```python
from build123d import *

# Parameters (mm, degrees)
PAD_DEPTH    = 20
SKETCH001_R  = 1.8
POCKET_DEPTH = 29.501


with BuildPart() as part:
    # Sketch → Pad (new body)
    with BuildSketch(Plane.XY):
        with BuildLine():
            ThreePointArc((-2.5, 17.825543), (0, -18), (2.5, 17.825543))
            Line((2.5, 32.062411), (2.5, 17.825543))
            Line((6.5, 32.062411), (2.5, 32.062411))
            Line((6.5, 22.062411), (6.5, 32.062411))
            ThreePointArc((-6.5, 22.062411), (0, -23), (6.5, 22.062411))
            Line((-6.5, 22.062411), (-6.5, 32.062411))
            Line((-6.5, 32.062411), (-2.5, 32.062411))
            Line((-2.5, 32.062411), (-2.5, 17.825543))
        make_face()
    extrude(amount=PAD_DEPTH)

    # Sketch001 → Pocket (cut, through all)
    with BuildSketch(Plane.YZ.offset(6.5)):
        with Locations((27.062411, 10)):
            Circle(SKETCH001_R)
    extrude(amount=-POCKET_DEPTH, mode=Mode.SUBTRACT)


solid = part.part
```
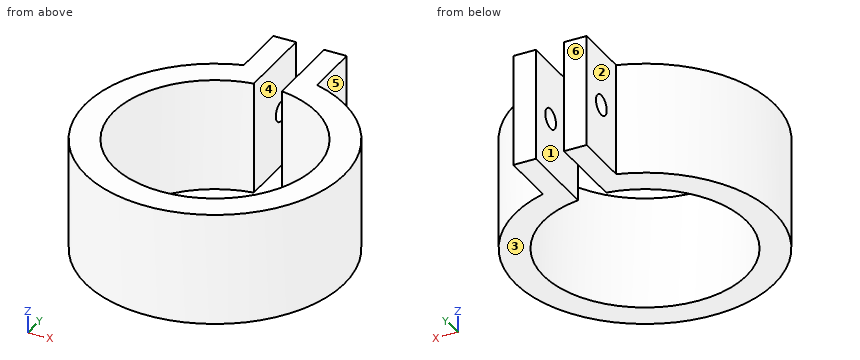
The model under review builds one solid part; all positions refer to its coordinate system, in mm. Face numbers are marked on the shaded views. A direction names the side the tool comes from. Give positions to 0.01 mm unless a question says otherwise; leave off trailing zeros. Write each loop counter-clockwise with the first axis right and the second up, starting at its lowest first coordinate (ties: lowest second). Pieces come first, ordered by that corner, then holes.
(1) Consider section D-D, the plane z = 5.75. Give the boundary of the cut face in (x, y).
(2) To check wall thickness, follow L1, parallel to X at y = 24, z = 15.5; L2, parallel to Y at x = 0, z = 6; L3, parallel to X at y = -13.5, z = 4.75. State the ranges of each line that lie inside material, in increasing order.
(3) Consider section C-C, the plane x = 10. Give the boundary of the cut face in (y, z), and give its area (3 significant figures).
(4) Consider section B-B, the plane y = 0. Give the boundary of the cut face in (x, z), and give its area (3 significant figures).
(5) Tool access review of the marked faces 1, 2 and 3: name each direction out of +Z, -Z, +X, -X, +Y, -Y from which nothing blocks a thin tool from reaching the whole face with its end or side.
(6) The part is to be moulded in two halves that separate along X. For the marked faces 4, 5 and 6, say which applies: released by +X, released by -X, zero draft, split by the parting line, or undercut.
(7) Consider section A-A, the plane z = 10. Give the boundary of the cut face in (x, y), and give its area (3 significant figures).
(8) For P1, Ø8, axis at y = 28, z = 8.5, coming from the -X side; P2, Ø6, axis at x = 14, z = 12.5, coming from the -Y side; P3, Ø1, axis at x = -12, z = 14, coming from the +Y side, all flat-tipped, find the tip position at first contact; note any pin that passes through.
Returned:
1. outline: (-6.5, 22.06) arc R23 ccw (long way) to (6.5, 22.06) - (6.5, 32.06) - (2.5, 32.06) - (2.5, 17.83) arc R18 cw (long way) to (-2.5, 17.83) - (-2.5, 32.06) - (-6.5, 32.06) - close
2. L1: x = -6.5 to -2.5, 2.5 to 6.5
2. L2: y = -23 to -18
2. L3: x = -18.62 to -11.91, 11.91 to 18.62
3. outline: (-20.71, 0) - (-14.97, 0) - (-14.97, 20) - (-20.71, 20) - close; (14.97, 0) - (20.71, 0) - (20.71, 20) - (14.97, 20) - close
3. area: 230 mm2
4. outline: (-23, 0) - (-18, 0) - (-18, 20) - (-23, 20) - close; (18, 0) - (23, 0) - (23, 20) - (18, 20) - close
4. area: 200 mm2
5. face 1: +Z, -Z, +Y
5. face 2: +Z, -Z, -X, +Y
5. face 3: -Z, +X, -X, +Y, -Y
6. face 4: undercut
6. face 5: released by +X
6. face 6: zero draft
7. outline: (-6.5, 22.06) arc R23 ccw (long way) to (6.5, 22.06) - (6.5, 25.26) - (2.5, 25.26) - (2.5, 17.83) arc R18 cw (long way) to (-2.5, 17.83) - (-2.5, 25.26) - (-6.5, 25.26) - close; (-6.5, 28.86) - (-2.5, 28.86) - (-2.5, 32.06) - (-6.5, 32.06) - close; (2.5, 28.86) - (6.5, 28.86) - (6.5, 32.06) - (2.5, 32.06) - close
7. area: 666 mm2
8. P1: stops at x = -6.5
8. P2: stops at y = -20.2
8. P3: stops at y = 19.92
